For this review, take the finished solid that the model builds, in its own axes (mm). Give positions to 0.01 mm unless a question says otherwise; leave off trailing zeros. Order: outer loops, then holes, each group sorted by start corner. A loop starts at its lowest first (then second) coordinate and runs counter-clockwise, first axis right, second up. Notation, with made-up numbers: (-3, -13.75) - (33, -13.75) arc R14 cw to (33, -0.75) - close; hole circle Ø6 at (85, -19). An arc over 180 degrees is marked (long way). Use a Markdown table: item, result. Add a question column.
1) We need section B-B on z = 25. Write out the cut boundary in (x, y), then the cut area to 3 significant figures.
2) We need section A-A on x = 0. Write out the cut boundary in (y, z).
3) Wall thickness on L1, parallel to Y at x = 0, z = 205.5; L2, parallel to Y at x = 4.25, z = 138; L3, parallel to X at y = 1.5, z = 92: over which ranges is each line inside the solid? List them lowest first.
4) Clearance check with flat-ended pins moving along their axes: P1, Ø3, axis at y = 0, z = 347.5, coming from the -X side; P2, Ø6, axis at x = -6.5, z = 167, coming from the +Y side; P3, Ø1, axis at x = -5, z = 85, coming from the -Y side; P4, Ø3, axis at x = -6.5, z = 141.5, coming from the -Y side. State where each tip first meets the part, or that it passes through.
```python
from build123d import *

# Parameters (mm, degrees)
SKETCH_1_R               = 9
SKETCH_1_R_2             = 6.25
EXTRUDE_1_DEPTH          = 400
SKETCH_2_R               = 1.75
CUT_EXTRUDE_1_DEPTH      = 10
CUT_EXTRUDE_1_DEPTH_BACK = 10


with BuildPart() as part:
    # ｽｹｯﾁ1 → ﾎﾞｽ - 押し出し1 (new body)
    with BuildSketch(Plane.XY):
        Circle(SKETCH_1_R)
        Circle(SKETCH_1_R_2, mode=Mode.SUBTRACT)
    extrude(amount=EXTRUDE_1_DEPTH)

    # ｽｹｯﾁ2 → ｶｯﾄ - 押し出し1 (cut, two sides)
    with BuildSketch(Plane(origin=(0, 0, 0), x_dir=(0, 0, -1), z_dir=(1, 0, 0))) as cut_extrude_1_sk:
        with Locations((-10, 0)):
            Circle(SKETCH_2_R)
        with Locations((-385, 0)):
            Circle(SKETCH_2_R)
        with Locations((-30, 0)):
            Circle(SKETCH_2_R)
        with Locations((-365, 0)):
            Circle(SKETCH_2_R)
        with Locations((-347.5, 0)):
            Circle(SKETCH_2_R)
        with Locations((-80, 0)):
            Circle(SKETCH_2_R)
    extrude(amount=CUT_EXTRUDE_1_DEPTH, mode=Mode.SUBTRACT)
    extrude(cut_extrude_1_sk.sketch, amount=-CUT_EXTRUDE_1_DEPTH_BACK, mode=Mode.SUBTRACT)


solid = part.part
```
Checked values:
| question | item | result |
|---|---|---|
| 1 | outline | circle Ø18 at (0, 0); hole circle Ø12.5 at (0, 0) |
| 1 | area | 132 mm² |
| 2 | outline | (-9, 0) - (-6.25, 0) - (-6.25, 400) - (-9, 400) - close; (6.25, 0) - (9, 0) - (9, 400) - (6.25, 400) - close |
| 3 | L1 | -9 to -6.25, 6.25 to 9 |
| 3 | L2 | -7.93 to -4.58, 4.58 to 7.93 |
| 3 | L3 | -8.87 to -6.07, 6.07 to 8.87 |
| 4 | P1 | through |
| 4 | P2 | y = 8.29 |
| 4 | P3 | y = -7.79 |
| 4 | P4 | y = -7.48 |
